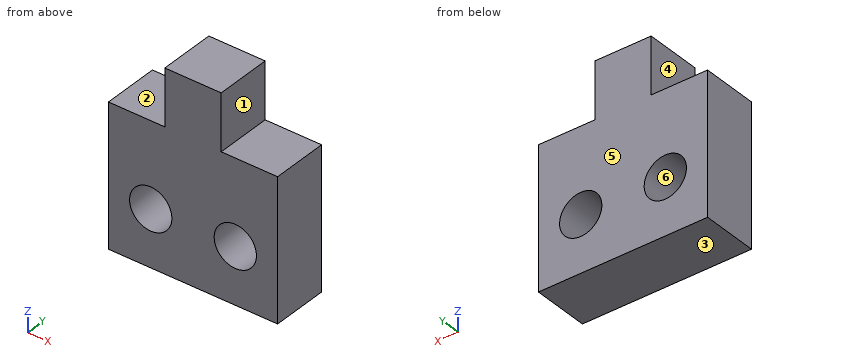
```python
from build123d import *

# Parameters (mm, degrees)
SKETCH1_W           = 12
SKETCH1_H           = 10
SKETCH1_W_2         = 4
SKETCH1_H_2         = 4
BOSS_EXTRUDE1_DEPTH = 4
SKETCH2_R           = 1.5
CUT_EXTRUDE1_DEPTH  = 12.532562595


with BuildPart() as part:
    # Sketch1 → Boss-Extrude1 (new body)
    with BuildSketch(Plane(origin=(0, 0, 0), x_dir=(1, 0, 0), z_dir=(0, 1, 0))):
        Rectangle(SKETCH1_W, SKETCH1_H)
        with Locations((0, -7)):
            Rectangle(SKETCH1_W_2, SKETCH1_H_2)
    extrude(amount=BOSS_EXTRUDE1_DEPTH)

    # Sketch2 → Cut-Extrude1 (cut, through all)
    with BuildSketch(Plane(origin=(0, 4, 0), x_dir=(1, 0, 0), z_dir=(0, 1, 0))):
        with Locations(Location((-3, 1, 0), (0, 0, 270))):
            Circle(SKETCH2_R)
        with Locations(Location((3, 1, 0), (0, 0, 270))):
            Circle(SKETCH2_R)
    extrude(amount=-CUT_EXTRUDE1_DEPTH, mode=Mode.SUBTRACT)


solid = part.part
```
Here's how the part is built. I have some questions about the finished solid (model axes, mm). Face numbers are marked on the shaded views. A direction names the side the tool comes from. Round coordinates to 2 decimals unless told otherwise and drop trailing zeros. Order: outer loops, then holes, each group sorted by start corner. A loop starts at its lowest first (then second) coordinate and runs counter-clockwise, first axis right, second up. Notation, with made-up numbers: M -8,11.5 L 11,11.5 A21 cw 11,35.5 Z; hole C 35.25,33 d11. An arc over 180 degrees is marked long. Answer as CSV lines item,"result".
Item 1: Imagine slicing it at D-D on x = 2.5. List the corners of the cut face in (y, z) for me, and give its area (3 significant figures).
From the geometry:
outline,"M 0,-5 L 4,-5 L 4,-2.41 L 0,-2.41 Z; M 0,0.41 L 4,0.41 L 4,5 L 0,5 Z"
area,"28.7 mm2"
Item 2: For pin 1 (2 mm diameter, centred on y = 1.5, z = 6.5, fed in from +X); pin 2 (1.2 mm diameter, centred on x = 3, y = 1.5, fed in from +Z), each with a flat end and sliding along its axis, tell me the tip position at first contact or that it passes through.
From the geometry:
pin 1,"x = 2"
pin 2,"z = 5"
Item 3: We'd pull the mould along X, two halves only. Please class the marked faces 4, 5 and 6: +X half, -X half, draft (parallel to the pull), parting line (faces both ways), or undercut.
From the geometry:
face 4,"-X half"
face 5,"draft"
face 6,"undercut"
Item 4: Imagine slicing it at B-B on z = -1. List the corners of the cut face in (x, y) for me.
From the geometry:
outline,"M -6,0 L -4.5,0 L -4.5,4 L -6,4 Z; M -1.5,0 L 1.5,0 L 1.5,4 L -1.5,4 Z; M 4.5,0 L 6,0 L 6,4 L 4.5,4 Z"
Item 5: Please list where these lines run through material, in increasing order: L1, parallel to X at y = 0.9, z = -1; L2, parallel to X at y = 2.25, z = -1.75; L3, parallel to X at y = 2.15, z = 7. Write a range as [from, to].
From the geometry:
L1,"[-6, -4.5], [-1.5, 1.5], [4.5, 6]"
L2,"[-6, -4.3], [-1.7, 1.7], [4.3, 6]"
L3,"[-2, 2]"
Item 6: Imagine slicing it at A-A on x = -3. List the corners of the cut face in (y, z) for me, and give its area (3 significant figures).
From the geometry:
outline,"M 0,-5 L 4,-5 L 4,-2.5 L 0,-2.5 Z; M 0,0.5 L 4,0.5 L 4,5 L 0,5 Z"
area,"28.0 mm2"
Item 7: Imagine slicing it at C-C on y = 2.35. List the corners of the cut face in (x, z) for me, and give its area (3 significant figures).
From the geometry:
outline,"M -6,-5 L 6,-5 L 6,5 L 2,5 L 2,9 L -2,9 L -2,5 L -6,5 Z; hole C -3,-1 d3; hole C 3,-1 d3"
area,"122 mm2"
Item 8: Which directions (+Z, -Z, +X, -X, +Y, -Y) give clear straight access to the entire face, cutting with the end or side of a thin tool? Please do the marked faces 1, 2 and 3.
From the geometry:
face 1,"+Z, +X, +Y, -Y"
face 2,"+Z, -X, +Y, -Y"
face 3,"-Z, +X, -X, +Y, -Y"
